```python
from build123d import *

# Parameters (mm, degrees)
F0_W          = 91.2663862109
F0_H          = 55.5524304509
F1_DEPTH      = 25.4
F2_W          = 31.717389822
F2_H          = 20.1121037826
F3_DEPTH      = 25.401
F4_R          = 9.4254777906
F5_DEPTH      = 76.2
F7_DEPTH      = 55.5534304509
F8_R          = 5.4499976888
F9_DEPTH      = 101.601
F10_W         = 10.9715163708
F10_H         = 9.965904057
F11_DEPTH     = 25.4
F12_T1_DEPTH  = 182.5524304509
F13_T4_DEPTH  = 98.5267601581
F13_T10_DEPTH = 98.5267601581
F13_T16_DEPTH = 98.5267601581
F13_T23_DEPTH = 98.5267601581
F13_T29_DEPTH = 98.5267601581
F13_T33_ANGLE = 163.70288589
F15_T4_DEPTH  = 53.5800548494
F15_T10_DEPTH = 53.5800548494
F15_T16_DEPTH = 53.5800548494
F17_D         = 4.2
F18_R         = 0.254


# Not quite as in the source:
# - a fillet or chamfer that OpenCascade refuses, or shapes differently, is made with other operations: its cross-section is extruded or revolved along the edge and cut away or added


with BuildPart() as f1:
    # F0 (on Top) → F1 (new body)
    with BuildSketch(Plane.XY):
        with Locations((-45.6331931055, -27.7762152255)):
            Rectangle(F0_W, F0_H)
    extrude(amount=F1_DEPTH)

    # F2 (on face) → F3 (cut, through all)
    with BuildSketch(Plane.XY.offset(25.4)):
        with Locations((-61.7938265204, -24.1600726731)):
            Rectangle(F2_W, F2_H)
    extrude(amount=-F3_DEPTH, mode=Mode.SUBTRACT)

    # F4 (on face) → F5 (join)
    with BuildSketch(Plane.XY.offset(25.4)):
        with Locations((-27.4883341044, -14.4118471071)):
            Circle(F4_R)
    extrude(amount=F5_DEPTH)

    # F6 (on face) → F7 (cut, through all)
    with BuildSketch(Plane.XZ.offset(55.5524304509)):
        Polygon((-39.0824638307, 12.301723844), (-39.0824638307, 18.5248410342), (-43.9478927691, 22.4048911381), (-50.0149834187, 21.0201172888), (-52.7150927741, 15.4132824391), (-50.0149834187, 9.8064475894), (-43.9478927691, 8.4216737401), align=None)
    extrude(amount=-F7_DEPTH, mode=Mode.SUBTRACT)

    # F8 (on face) → F9 (cut, through all)
    with BuildSketch(Plane.XY.offset(101.6)):
        with Locations((-27.4883341044, -14.4118471071)):
            Circle(F8_R)
    extrude(amount=-F9_DEPTH, mode=Mode.SUBTRACT)

    # F10 (on face) → F11 (join)
    with BuildSketch(Plane.XY.offset(25.4)):
        with Locations((-25.7194377482, -40.6495332718)):
            Rectangle(F10_W, F10_H)
    extrude(amount=F11_DEPTH)

    # F12: fillet of radius 25.4 on 1 edges, made by hand

    # F12_s2 → F12_t1 (cut)
    with BuildSketch(Plane.XZ.offset(-63.5)):
        with BuildLine():
            ThreePointArc((-91.2663862109, 0), (-83.8268984531, 17.9605122421), (-65.8663862109, 25.4))
            Line((-65.8663862109, 25.4), (-91.2663862109, 25.4))
            Line((-91.2663862109, 25.4), (-91.2663862109, 0))
        make_face()
    extrude(amount=F12_T1_DEPTH, mode=Mode.SUBTRACT)

    # F13: chamfer of 12.7 on 1 edges, made by hand


with BuildPart() as f13_tool2:
    # F13_s3 → F13_t4 (new body)
    with BuildSketch(Plane.YZ.offset(-65.8663862109)):
        Polygon((-55.5524304509, 12.7), (-42.8524304509, 25.4), (-55.5524304509, 25.4), align=None)
    extrude(amount=F13_T4_DEPTH)

    split(bisect_by=Plane.YZ.offset(-31.2051959336), keep=Keep.BOTTOM)

    split(bisect_by=Plane.XZ.offset(45.6324853003), keep=Keep.TOP)


with BuildPart() as f1_1:
    add(f1.part)

    # F13_t1: cut F13_tool2
    add(f13_tool2.part, mode=Mode.SUBTRACT)


with BuildPart() as f13_tool8:
    # F13_s9 → F13_t10 (new body)
    with BuildSketch(Plane.YZ.offset(-65.8663862109)):
        Polygon((-55.5524304509, 12.7), (-42.8524304509, 25.4), (-55.5524304509, 25.4), align=None)
    extrude(amount=F13_T10_DEPTH)

    split(bisect_by=Plane.YZ.offset(-31.2051959336), keep=Keep.BOTTOM)

    split(bisect_by=Plane.XZ.offset(45.6324853003), keep=Keep.BOTTOM)


with BuildPart() as f1_2:
    add(f1_1.part)

    # F13_t7: cut F13_tool8
    add(f13_tool8.part, mode=Mode.SUBTRACT)


with BuildPart() as f13_tool14:
    # F13_s15 → F13_t16 (new body)
    with BuildSketch(Plane.YZ.offset(-65.8663862109)):
        Polygon((-55.5524304509, 12.7), (-42.8524304509, 25.4), (-55.5524304509, 25.4), align=None)
    extrude(amount=F13_T16_DEPTH)

    split(bisect_by=Plane.YZ.offset(-20.2336795628), keep=Keep.BOTTOM)

    split(bisect_by=Plane.YZ.offset(-31.2051959336), keep=Keep.TOP)

    split(bisect_by=Plane.XZ.offset(45.6324853003), keep=Keep.TOP)


with BuildPart() as f1_3:
    add(f1_2.part)

    # F13_t13: cut F13_tool14
    add(f13_tool14.part, mode=Mode.SUBTRACT)


with BuildPart() as f13_tool21:
    # F13_s22 → F13_t23 (new body)
    with BuildSketch(Plane.YZ.offset(-65.8663862109)):
        Polygon((-55.5524304509, 12.7), (-42.8524304509, 25.4), (-55.5524304509, 25.4), align=None)
    extrude(amount=F13_T23_DEPTH)

    split(bisect_by=Plane.YZ.offset(-20.2336795628), keep=Keep.TOP)

    split(bisect_by=Plane.XZ.offset(45.6324853003), keep=Keep.TOP)


with BuildPart() as f1_4:
    add(f1_3.part)

    # F13_t20: cut F13_tool21
    add(f13_tool21.part, mode=Mode.SUBTRACT)


with BuildPart() as f13_tool27:
    # F13_s28 → F13_t29 (new body)
    with BuildSketch(Plane.YZ.offset(-65.8663862109)):
        Polygon((-55.5524304509, 12.7), (-42.8524304509, 25.4), (-55.5524304509, 25.4), align=None)
    extrude(amount=F13_T29_DEPTH)

    split(bisect_by=Plane.YZ.offset(-20.2336795628), keep=Keep.TOP)

    split(bisect_by=Plane.XZ.offset(45.6324853003), keep=Keep.BOTTOM)


with BuildPart() as f1_5:
    add(f1_4.part)

    # F13_t26: cut F13_tool27
    add(f13_tool27.part, mode=Mode.SUBTRACT)

    # F13_s32 → F13_t33 (revolve, cut)
    with BuildSketch(Plane(origin=(-60.6796278509, 0, 17.7406473118), x_dir=(0, 1, 0), z_dir=(0.9598194275, 0, -0.2806183648))):
        Polygon((-42.8524304509, -43.8833175952), (-55.5524304509, -31.1833175952), (-55.5524304509, -43.8833175952), align=None)
    revolve(axis=Axis((-65.8663862109, -55.5524304509, 0), (0, 1, 0)), revolution_arc=F13_T33_ANGLE, mode=Mode.SUBTRACT)

    # F14: chamfer of 5.08 on 1 edges, made by hand

    # F14_s1 → F14_t2 (revolve, cut)
    with BuildSketch(Plane.XZ.offset(14.4118471071)):
        Polygon((-23.1428563138, 101.6), (-18.0628563138, 96.52), (-18.0628563138, 101.6), align=None)
    revolve(axis=Axis((-27.4883341044, -14.4118471071, 101.6), (0, 0, 1)), mode=Mode.SUBTRACT)

    # F15: fillet of radius 5.08 on 1 edges, made by hand


with BuildPart() as f15_tool2:
    # F15_s3 → F15_t4 (new body)
    with BuildSketch(Plane.XY.offset(63.5)):
        with BuildLine():
            ThreePointArc((-20.2336795628, -40.5524853003), (-21.7215771144, -44.1445877487), (-25.3136795628, -45.6324853003))
            Line((-25.3136795628, -45.6324853003), (-20.2336795628, -45.6324853003))
            Line((-20.2336795628, -45.6324853003), (-20.2336795628, -40.5524853003))
        make_face()
    extrude(amount=-F15_T4_DEPTH)

    split(bisect_by=Plane.XY.offset(25.4), keep=Keep.TOP)

    split(bisect_by=Plane(origin=(0, -34.1262152254, 34.1262152254), x_dir=(1, 0, 0), z_dir=(0, -0.7071067812, 0.7071067812)), keep=Keep.TOP)


with BuildPart() as f1_6:
    add(f1_5.part)

    # F15_t1: cut F15_tool2
    add(f15_tool2.part, mode=Mode.SUBTRACT)


with BuildPart() as f15_tool8:
    # F15_s9 → F15_t10 (new body)
    with BuildSketch(Plane.XY.offset(63.5)):
        with BuildLine():
            ThreePointArc((-20.2336795628, -40.5524853003), (-21.7215771144, -44.1445877487), (-25.3136795628, -45.6324853003))
            Line((-25.3136795628, -45.6324853003), (-20.2336795628, -45.6324853003))
            Line((-20.2336795628, -45.6324853003), (-20.2336795628, -40.5524853003))
        make_face()
    extrude(amount=-F15_T10_DEPTH)

    split(bisect_by=Plane.XY.offset(25.4), keep=Keep.BOTTOM)

    split(bisect_by=Plane(origin=(0, -34.1262152255, 34.1262152254), x_dir=(1, 0, 0), z_dir=(0, -0.7071067812, 0.7071067812)), keep=Keep.TOP)


with BuildPart() as f1_7:
    add(f1_6.part)

    # F15_t7: cut F15_tool8
    add(f15_tool8.part, mode=Mode.SUBTRACT)


with BuildPart() as f15_tool14:
    # F15_s15 → F15_t16 (new body)
    with BuildSketch(Plane.XY.offset(63.5)):
        with BuildLine():
            ThreePointArc((-20.2336795628, -40.5524853003), (-21.7215771144, -44.1445877487), (-25.3136795628, -45.6324853003))
            Line((-25.3136795628, -45.6324853003), (-20.2336795628, -45.6324853003))
            Line((-20.2336795628, -45.6324853003), (-20.2336795628, -40.5524853003))
        make_face()
    extrude(amount=-F15_T16_DEPTH)

    split(bisect_by=Plane.XY.offset(25.4), keep=Keep.TOP)

    split(bisect_by=Plane(origin=(0, -34.1262152255, 34.1262152254), x_dir=(1, 0, 0), z_dir=(0, 0.7071067812, -0.7071067812)), keep=Keep.TOP)


with BuildPart() as f1_8:
    add(f1_7.part)

    # F15_t13: cut F15_tool14
    add(f15_tool14.part, mode=Mode.SUBTRACT)

    # F17 (through all)
    with Locations(Plane.XY.offset(25.4)):
        with Locations((-37.6806370914, -34.2161245644), (-43.5164868832, -5.5432366207)):
            Hole(F17_D / 2)

    # F18
    f18_edges = [f1_8.edges().sort_by_distance(p)[0] for p in [
        (-83.826898, 0, 17.960512),
    ]]
    fillet(f18_edges, radius=F18_R)


solid = f1_8.part
```
Work out the finished part from the listing and answer in its coordinate system (mm). A direction names the side the tool comes from. Give positions to 0.01 mm unless a question says otherwise; leave off trailing zeros. Loops run counter-clockwise (first coordinate to the right, second up) from the corner with the lowest first, then second, coordinate; pieces in that order, holes last. Notation, with made-up numbers: (21.5, 80.25) -> (56.5, 80.25) arc R12 cw to (56.5, 92.25) -> close; hole circle Ø4 at (27.25, 43). An arc over 180 degrees is marked (long way). Use CSV: the item, a comma, the result in double quotes.
1. The part is cut by section C-C (z = 40.5). Write down the section's boundary in (x, y), then the cut area to 3 significant figures.
Found:
outline,"circle Ø18.85 at (-27.49, -14.41); (-31.21, -45.63) -> (-25.31, -45.63) arc R5.08 ccw to (-20.23, -40.55) -> (-20.23, -35.67) -> (-31.21, -35.67) -> close; hole circle Ø10.9 at (-27.49, -14.41)"
area,"290 mm^2"
2. The part is cut by section B-B (x = -56.5). Write down the section's boundary in (y, z), then the cut area to 3 significant figures.
Found:
outline,"(-55.55, 0) -> (-34.22, 0) -> (-34.22, 25.4) -> (-42.85, 25.4) -> (-55.55, 12.7) -> close; (-14.1, 0) -> (0, 0) -> (0, 25.15) arc R0.25 ccw to (-0.25, 25.4) -> (-14.1, 25.4) -> close"
area,"820 mm^2"
3. Straight lines are drawn through the part: line 1 (X direction, y = -14.5, z = 45); line 2 (X direction, y = -18.5, z = 14); line 3 (Y direction, x = -30, z = 33). For each, find the intervals that lie inside material, in ascending order.
Found:
line 1,"-36.91 to -32.94, -22.04 to -18.06"
line 2,"-87.06 to -77.65, -39.08 to -31.09, -23.88 to 0"
line 3,"-45.63 to -35.67, -23.5 to -19.25, -9.58 to -5.33"
4. The part is cut by section D-D (y = -12). State how many separate pieces and enclosed holes the cut face has, then the cut area to 3 significant figures.
Found:
separate pieces,"2"
enclosed holes,"1"
area,"2,410 mm^2"
5. A tool of negligible diameter and unlimited length cuts with its end or side. For faces 1 (the flat face through (-26, -41, 50.8)), 2 (the flat face through (-39.082, -44, 15)), 3 (the flat face through (-26, -35.667, 38)), 4 (the cylindrical face through (-18.5, -11.58, 60.46)), from which of +Z, -Z, +X, -X, +Y, -Y can it reach the whole face along a straight path? Write none if from no direction.
Found:
face 1,"+Z, +X, -X, -Y"
face 2,"+Y, -Y"
face 3,"+Z, +X, -X"
face 4,"+Z"
6. Flat-ended cylindrical pins translate along their axes: pin 1 Ø10 at (y, z) = (-22.5, 3) entering from -X; pin 2 Ø4 at (x, y) = (-43.52, -5.54) entering from +Z; pin 3 Ø1.5 at (x, y) = (-56, -13.5) entering from +Z; pin 4 Ø1 at (y, z) = (-29, 24.5) entering from -X. Find the tip coordinate at first contact, or state that the pin passes through.
Found:
pin 1,"x = -91.27"
pin 2,"through"
pin 3,"z = 25.4"
pin 4,"x = -45.94"
7. The part is cut by section A-A (y = -26). Write down the section's boundary in (x, z), then the cut area to 3 significant figures.
Found:
outline,"(-91.27, 0) -> (-77.65, 0) -> (-77.65, 22.5) arc R25.4 ccw to start; (-45.94, 0) -> (0, 0) -> (0, 25.4) -> (-45.94, 25.4) -> (-45.94, 21.95) -> (-43.95, 22.4) -> (-39.08, 18.52) -> (-39.08, 12.3) -> (-43.95, 8.42) -> (-45.94, 8.88) -> close"
area,"1,310 mm^2"
8. The mould has two halves that part along Z. Classify faces 5 (the flat face through (-33, -26, 25.4)), 6 (the cylindrical face through (-32.933, -14.172, 50.951)), 7 (the flat face through (-51.346, -41.589, 18.256)), 8 (the flat face through (-41.481, -25.212, 20.438)): +Z half, -Z half, draft (parallel to the pull), parting line (faces both ways), or undercut.
Found:
face 5,"+Z half"
face 6,"draft"
face 7,"undercut"
face 8,"undercut"
